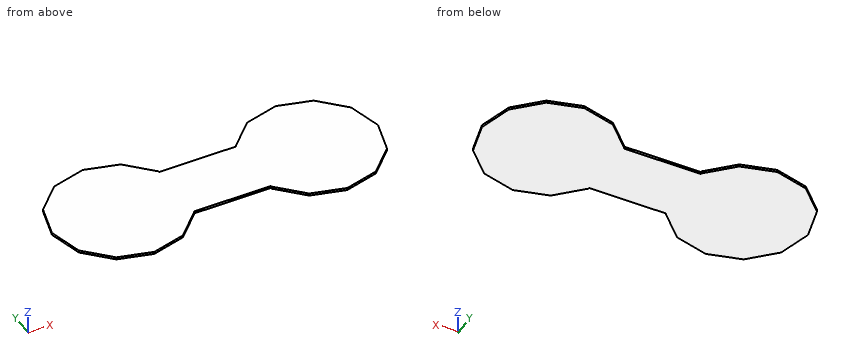
from build123d import *

# Parameters (mm, degrees)
F1_DEPTH = 12.7
F3_W     = 1066.8
F3_H     = 355.6
F4_DEPTH = 12.7


with BuildPart() as f1:
    # F0 (on Top) → F1 (new body)
    with BuildSketch(Plane.XY):
        Polygon((184.072105, 318.822238), (0, 368.14421), (-184.072105, 318.822238), (-318.822238, 184.072105), (-368.14421, 0), (-318.822238, -184.072105), (-184.072105, -318.822238), (0, -368.14421), (184.072105, -318.822238), (318.822238, -184.072105), (368.14421, 0), (318.822238, 184.072105), align=None)
    extrude(amount=F1_DEPTH)



with BuildPart() as f2_1:
    # F2: copy of F1
    add(f1.part.moved(Location((1066.8, 0, 0))))


with BuildPart() as f1_1:
    add(f1.part)

    add(f2_1.part)  # F4 merges F2_1
    # F3 (on face) → F4 (join, through all)
    with BuildSketch(Plane.XY.offset(12.7)):
        with Locations((533.4, 0)):
            Rectangle(F3_W, F3_H)
    extrude(amount=-F4_DEPTH)


solid = f1_1.part
Check sheet for the modelled part. Datum: model origin and axes. Units: mm. Coordinates: 2 decimals unless noted, no trailing zeros. Loops run counter-clockwise (first coordinate to the right, second up) from the corner with the lowest first, then second, coordinate; pieces in that order, holes last. Notation, with made-up numbers: (40.5, -27.5) -> (67.5, -27.5) arc R24 ccw to (67.5, -16.5) -> close; hole circle Ø6 at (-25.5, -38). An arc over 180 degrees is marked (long way). Answer in a Markdown table with one row per item.
1. Sectioned sample at B-B, the plane z = 7. Record the boundary of the cut face in (x, y).
Check values:
| item | result |
|---|---|
| outline | (-368.14, 0) -> (-318.82, -184.07) -> (-184.07, -318.82) -> (0, -368.14) -> (184.07, -318.82) -> (318.82, -184.07) -> (320.5, -177.8) -> (746.3, -177.8) -> (747.98, -184.07) -> (882.73, -318.82) -> (1066.8, -368.14) -> (1250.87, -318.82) -> (1385.62, -184.07) -> (1434.94, 0) -> (1385.62, 184.07) -> (1250.87, 318.82) -> (1066.8, 368.14) -> (882.73, 318.82) -> (747.98, 184.07) -> (746.3, 177.8) -> (320.5, 177.8) -> (318.82, 184.07) -> (184.07, 318.82) -> (0, 368.14) -> (-184.07, 318.82) -> (-318.82, 184.07) -> close |
2. Sectioned sample at A-A, the plane y = 299.5. Record the boundary of the cut face in (x, z), then the cut area to 3 significant figures.
Check values:
| item | result |
|---|---|
| outline | (-203.39, 0) -> (203.39, 0) -> (203.39, 12.7) -> (-203.39, 12.7) -> close; (863.41, 0) -> (1270.19, 0) -> (1270.19, 12.7) -> (863.41, 12.7) -> close |
| area | 10,300 mm2 |
3. Material ranges on line 1 along Y through (x, z) = (366, 11.5); line 2 along X through (y, z) = (241, 5.25); line 3 along X through (y, z) = (-248, 10), recorded low to high. Write a range as [from, to].
Check values:
| item | result |
|---|---|
| line 1 | y = [-177.8, 177.8] |
| line 2 | x = [-261.89, 261.89], [804.91, 1328.69] |
| line 3 | x = [-254.89, 254.89], [811.91, 1321.69] |
4. Go/stop test with flat-tipped pins: pin 1 (1.5 mm diameter, centred on y = 241, z = 4, fed in from +X); pin 2 (4 mm diameter, centred on x = 444.5, z = 5.5, fed in from +Y); pin 3 (3 mm diameter, centred on x = 364.5, y = 79.5, fed in from -Z); pin 4 (3 mm diameter, centred on x = 507, z = 11, fed in from -Y). Record where each tip stops, or that it passes through.
Check values:
| item | result |
|---|---|
| pin 1 | stops at x = 1329.44 |
| pin 2 | stops at y = 177.8 |
| pin 3 | stops at z = 0 |
| pin 4 | stops at y = -177.8 |
5. Sectioned sample at C-C, the plane x = 531. Record the boundary of the cut face in (y, z), then the cut area to 3 significant figures.
Check values:
| item | result |
|---|---|
| outline | (-177.8, 0) -> (177.8, 0) -> (177.8, 12.7) -> (-177.8, 12.7) -> close |
| area | 4,520 mm2 |
6. Sectioned sample at D-D, the plane y = 151.5. Record the boundary of the cut face in (x, z).
Check values:
| item | result |
|---|---|
| outline | (-327.55, 0) -> (1394.35, 0) -> (1394.35, 12.7) -> (-327.55, 12.7) -> close |
